```python
from build123d import *

# Parameters (mm, degrees)
F0_R     = 1.4
F0_R_2   = 1.7
F0_R_3   = 9
F1_DEPTH = 1.2
F2_R     = 1.4
F2_R_2   = 1.7
F2_R_3   = 11.35
F3_DEPTH = 3.4
F4_R     = 0.8


with BuildPart() as f1:
    # F0 (on Right) → F1 (new body)
    with BuildSketch(Plane.YZ):
        with BuildLine():
            Line((36.315416, 6.963249), (56.281398, 16.202273))
            Line((56.281398, 16.202273), (55.69346, 17.472835))
            Line((55.69346, 17.472835), (75.164664, 26.482906))
            ThreePointArc((75.164664, 26.482906), (78.467758, 27.367196), (81.875669, 27.086954))
            Line((81.875669, 27.086954), (102.642848, 21.698686))
            Line((102.642848, 21.698686), (102.291245, 20.343557))
            Line((102.291245, 20.343557), (123.586134, 14.818369))
            Line((123.586134, 14.818369), (123.937737, 16.173498))
            Line((123.937737, 16.173498), (135.389363, 13.202251))
            ThreePointArc((135.389363, 13.202251), (137.676185, 12.296386), (139.672705, 10.859704))
            Line((139.672705, 10.859704), (148.352908, 2.820916))
            Line((148.352908, 2.820916), (147.401638, 1.793743))
            Line((147.401638, 1.793743), (163.542923, -13.154799))
            Line((163.542923, -13.154799), (164.494194, -12.127626))
            ThreePointArc((164.494194, -12.127626), (165.178749, -8.371866), (163.889187, -4.778626))
            ThreePointArc((163.889187, -4.778626), (80.505559, 44.237166), (-10.894182, 12.591239))
            Line((-10.894182, 12.591239), (-13.722609, 15.419666))
            Line((-13.722609, 15.419666), (-12.874081, 16.268194))
            ThreePointArc((-12.874081, 16.268194), (-16.268194, 16.268194), (-16.268194, 12.874081))
            Line((-16.268194, 12.874081), (-15.419666, 13.722609))
            Line((-15.419666, 13.722609), (-12.591239, 10.894182))
            ThreePointArc((-12.591239, 10.894182), (-11.773328, -11.773328), (10.894182, -12.591239))
            Line((10.894182, -12.591239), (13.722609, -15.419666))
            Line((13.722609, -15.419666), (12.874081, -16.268194))
            ThreePointArc((12.874081, -16.268194), (16.268194, -16.268194), (16.268194, -12.874081))
            Line((16.268194, -12.874081), (15.419666, -13.722609))
            Line((15.419666, -13.722609), (12.591239, -10.894182))
            ThreePointArc((12.591239, -10.894182), (14.365147, -8.418138), (15.65831, -5.660373))
            Line((15.65831, -5.660373), (16.240046, -4.051116))
            ThreePointArc((16.240046, -4.051116), (18.274186, -0.692085), (21.44488, 1.624707))
            Line((21.44488, 1.624707), (35.727478, 8.233812))
            Line((35.727478, 8.233812), (36.315416, 6.963249))
        make_face()
        with Locations((-9.86414, -9.86414)):
            Circle(F0_R, mode=Mode.SUBTRACT)
        with Locations((9.86414, -9.86414)):
            Circle(F0_R_2, mode=Mode.SUBTRACT)
        Circle(F0_R_3, mode=Mode.SUBTRACT)
        with Locations((-9.86414, 9.86414)):
            Circle(F0_R, mode=Mode.SUBTRACT)
        with Locations((9.86414, 9.86414)):
            Circle(F0_R_2, mode=Mode.SUBTRACT)
    extrude(amount=F1_DEPTH)

    # F2 (on face) → F3 (join)
    with BuildSketch(Plane.YZ.offset(1.2)):
        with BuildLine():
            Line((102.291245, 20.343557), (123.586134, 14.818369))
            Line((123.586134, 14.818369), (123.937737, 16.173498))
            Line((123.937737, 16.173498), (135.389363, 13.202251))
            ThreePointArc((135.389363, 13.202251), (137.676185, 12.296386), (139.672705, 10.859704))
            Line((139.672705, 10.859704), (148.352908, 2.820916))
            Line((148.352908, 2.820916), (147.401638, 1.793743))
            Line((147.401638, 1.793743), (163.542923, -13.154799))
            Line((163.542923, -13.154799), (164.494194, -12.127626))
            ThreePointArc((164.494194, -12.127626), (165.178749, -8.371866), (163.889187, -4.778626))
            ThreePointArc((163.889187, -4.778626), (80.505559, 44.237166), (-10.894182, 12.591239))
            Line((-10.894182, 12.591239), (-13.722609, 15.419666))
            Line((-13.722609, 15.419666), (-12.874081, 16.268194))
            ThreePointArc((-12.874081, 16.268194), (-16.268194, 16.268194), (-16.268194, 12.874081))
            Line((-16.268194, 12.874081), (-15.419666, 13.722609))
            Line((-15.419666, 13.722609), (-12.591239, 10.894182))
            ThreePointArc((-12.591239, 10.894182), (-11.773328, -11.773328), (10.894182, -12.591239))
            Line((10.894182, -12.591239), (13.722609, -15.419666))
            Line((13.722609, -15.419666), (12.874081, -16.268194))
            ThreePointArc((12.874081, -16.268194), (16.268194, -16.268194), (16.268194, -12.874081))
            Line((16.268194, -12.874081), (15.419666, -13.722609))
            Line((15.419666, -13.722609), (12.591239, -10.894182))
            ThreePointArc((12.591239, -10.894182), (14.365147, -8.418138), (15.65831, -5.660373))
            Line((15.65831, -5.660373), (16.240046, -4.051116))
            ThreePointArc((16.240046, -4.051116), (18.274186, -0.692085), (21.44488, 1.624707))
            Line((21.44488, 1.624707), (35.727478, 8.233812))
            Line((35.727478, 8.233812), (36.315416, 6.963249))
            Line((36.315416, 6.963249), (56.281398, 16.202273))
            Line((56.281398, 16.202273), (55.69346, 17.472835))
            Line((55.69346, 17.472835), (75.164664, 26.482906))
            ThreePointArc((75.164664, 26.482906), (78.467758, 27.367196), (81.875669, 27.086954))
            Line((81.875669, 27.086954), (102.642848, 21.698686))
            Line((102.642848, 21.698686), (102.291245, 20.343557))
        make_face()
        with Locations((-9.86414, -9.86414)):
            Circle(F2_R, mode=Mode.SUBTRACT)
        with Locations((9.86414, -9.86414)):
            Circle(F2_R_2, mode=Mode.SUBTRACT)
        Circle(F2_R_3, mode=Mode.SUBTRACT)
        with Locations((-9.86414, 9.86414)):
            Circle(F2_R, mode=Mode.SUBTRACT)
        with Locations((9.86414, 9.86414)):
            Circle(F2_R_2, mode=Mode.SUBTRACT)
    extrude(amount=F3_DEPTH)

    # F4
    f4_edges = [f1.edges().sort_by_distance(p)[0] for p in [
        (2.3, 12.874081, -16.268194),
        (2.3, -16.268194, 12.874081),
        (2.3, -12.874081, 16.268194),
        (2.3, 10.894182, -12.591239),
        (2.3, 12.591239, -10.894182),
        (2.3, 16.268194, -12.874081),
        (2.3, -10.894182, 12.591239),
        (2.3, -12.591239, 10.894182),
    ]]
    fillet(f4_edges, radius=F4_R)


solid = f1.part
```
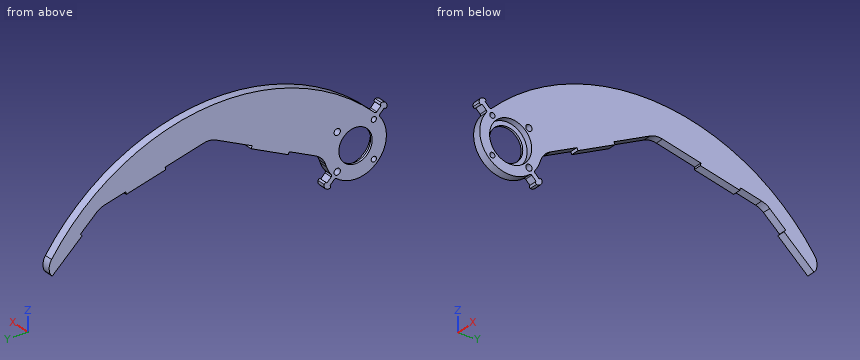
Check sheet for the modelled part. Datum: model origin and axes. Units: mm. Coordinates: 2 decimals unless noted, no trailing zeros. Order: outer loops, then holes, each group sorted by start corner. A loop starts at its lowest first (then second) coordinate and runs counter-clockwise, first axis right, second up. Notation, with made-up numbers: (81.5, 10) -> (115.5, 10) arc R9 cw to (115.5, 17) -> close; hole circle Ø2 at (1.5, 36.25). An arc over 180 degrees is marked (long way). Write item = value, one per line. Start each with the question number.
1) Material ranges on L1, parallel to Y at x = 0.2, z = 4.5; L2, parallel to Y at x = 2.6, z = -0.5; L3, parallel to Z at x = 3.85, y = 0, recorded low to high.
2) Cross-section at B-B (z = 0). Enter the section's corners in (x, y), then the cut area to 3 significant figures.
3) Go/stop test with flat-tipped pins: P1, Ø20.5, axis at y = 0, z = 0, coming from the +X side; P2, Ø3, axis at y = 9.86, z = 9.86, coming from the -X side; P3, Ø1.5, axis at x = 0.5, y = 71, coming from the +Z side; P4, Ø2, axis at x = 1.5, z = 27.5, coming from the -Y side. Record where each tip stops, or that it passes through.
4) Cross-section at A-A (y = 0). Enter the section's corners in (x, z), then the cut area to 3 significant figures.
5) Cross-section at C-C (x = 3.65). State how many separate pieces and enclosed holes the cut face has, then the cut area to 3 significant figures.
6) Cross-section at D-D (z = 34.5). Enter the section's corners in (x, y).
Ans:
q1.L1 = -16.03 to -7.79, 7.79 to 27.66, 146.54 to 156.72
q1.L2 = -16.64 to -11.34, 11.34 to 18.46, 149.88 to 160.77
q1.L3 = -16.65 to -11.35, 11.35 to 21.84
q2.outline = (0, -16.65) -> (4.6, -16.65) -> (4.6, -11.35) -> (1.2, -11.35) -> (1.2, -9) -> (0, -9) -> close; (0, 9) -> (1.2, 9) -> (1.2, 11.35) -> (4.6, 11.35) -> (4.6, 18.97) -> (0, 18.97) -> close; (0, 149.34) -> (4.6, 149.34) -> (4.6, 160.39) -> (0, 160.39) -> close
q2.area = 116 mm²
q3.P1 = 1.2
q3.P2 = through
q3.P3 = 44.8
q3.P4 = 6.72
q4.outline = (0, -16.65) -> (4.6, -16.65) -> (4.6, -11.35) -> (1.2, -11.35) -> (1.2, -9) -> (0, -9) -> close; (0, 9) -> (1.2, 9) -> (1.2, 11.35) -> (4.6, 11.35) -> (4.6, 21.84) -> (0, 21.84) -> close
q4.area = 78.3 mm²
q5.separate_pieces = 1
q5.enclosed_holes = 5
q5.area = 3,750 mm²
q6.outline = (0, 21.43) -> (4.6, 21.43) -> (4.6, 116.76) -> (0, 116.76) -> close
